Verification items for this drawing (mm, ordinates from the low corner). A direction names the side the tool comes from. Round coordinates to 2 decimals unless told otherwise and drop trailing zeros. Write each loop counter-clockwise with the first axis right and the second up, starting at its lowest first coordinate (ties: lowest second). Pieces come first, ordered by that corner, then holes. Notation, with made-up numbers: (52, 4.5) -> (88, 4.5) arc R35 ccw to (88, 37.5) -> close; hole circle Ø7 at (55.5, 24). An arc over 180 degrees is marked (long way). One line per question, with ' | ' between items.
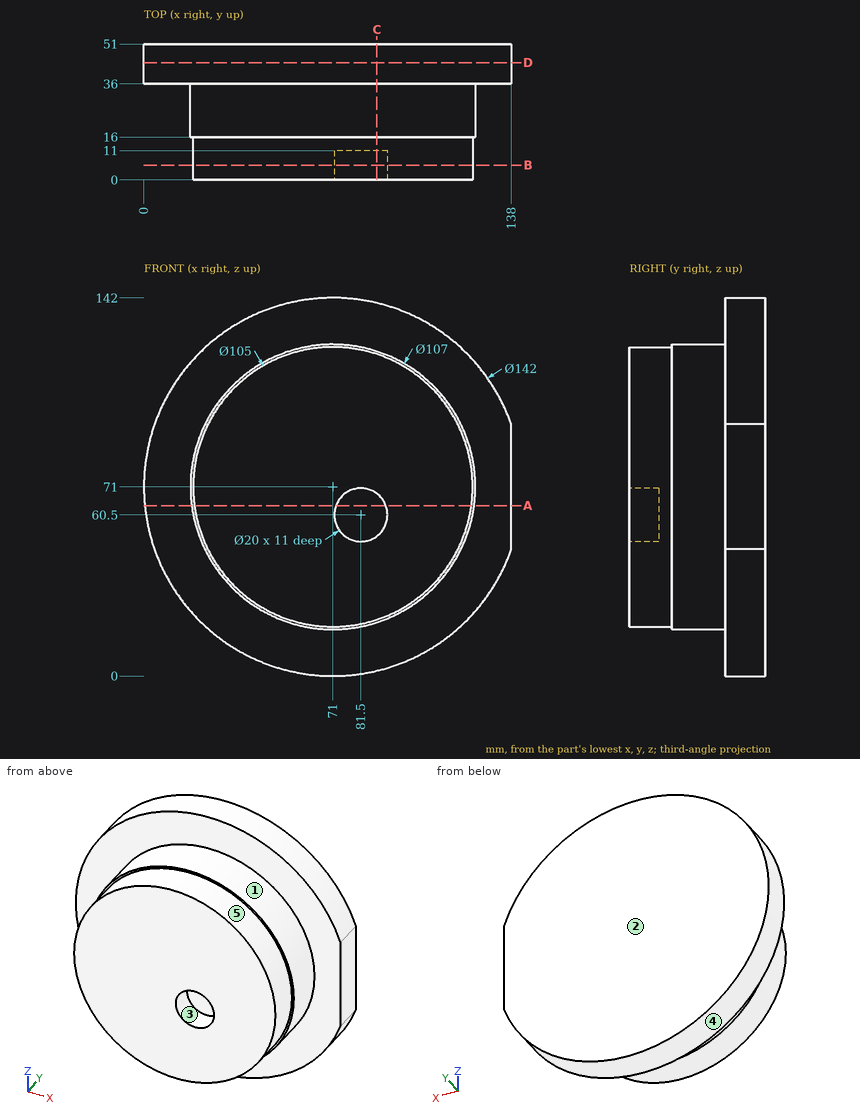
(1) Sectioned sample at A-A on z = 64. Record the cut outline in (x, y).
Resolved:
outline: (0.35, 36) -> (17.96, 36) -> (17.96, 16) -> (18.97, 16) -> (18.97, 0) -> (72.13, 0) -> (72.13, 11) -> (90.87, 11) -> (90.87, 0) -> (123.03, 0) -> (123.03, 16) -> (124.04, 16) -> (124.04, 36) -> (138, 36) -> (138, 51) -> (0.35, 51) -> close
(2) Material ranges on line 1 (X direction, y = 6.75, z = 60.5); line 2 (Y direction, x = 59, z = 6); line 3 (Z direction, x = 81.5, y = 2.5), recorded low to high.
Resolved:
line 1: x = 19.56 to 71.5, 91.5 to 122.44 | line 2: y = 36 to 51 | line 3: z = 19.56 to 50.5, 70.5 to 122.44
(3) Draft check along Z on the marked faces 1, 2 and 3. Enter one of: +Z half, -Z half, draft (parallel to the pull), parting line (faces both ways), or undercut.
Resolved:
face 1: parting line | face 2: draft | face 3: undercut
(4) Sectioned sample at D-D on y = 44. Record the cut outline in (x, z), then the cut area to 3 significant figures.
Resolved:
outline: (138, 47.51) -> (138, 94.49) arc R71 ccw (long way) to start | area: 15,700 mm2
(5) Go/stop test with flat-tipped pins: pin 1 (3 mm diameter, centred on x = 57.5, y = 35.5, fed in from +Z); pin 2 (10 mm diameter, centred on x = 31.5, y = 7, fed in from -Z); pin 3 (12 mm diameter, centred on y = 20, z = 32, fed in from +X). Record where each tip stops, or that it passes through.
Resolved:
pin 1: stops at z = 140.96 | pin 2: stops at z = 31.43 | pin 3: stops at x = 113.11
(6) Sectioned sample at B-B on y = 5.5. Record the cut outline in (x, z).
Resolved:
outline: circle Ø105 at (71, 71); hole circle Ø20 at (81.5, 60.5)
(7) Access from +Z, -Z, +X, -X, +Y, -Y to the whole of each face (thin tool, end or side, straight path). Record for the marked faces 4 and 5.
Resolved:
face 4: +Y, -Y | face 5: -Y
(8) Sectioned sample at C-C on x = 87.5. Record the cut outline in (y, z), then the cut area to 3 significant figures.
Resolved:
outline: (0, 21.16) -> (16, 21.16) -> (16, 20.11) -> (36, 20.11) -> (36, 1.94) -> (51, 1.94) -> (51, 140.06) -> (36, 140.06) -> (36, 121.89) -> (16, 121.89) -> (16, 120.84) -> (0, 120.84) -> (0, 68.5) -> (11, 68.5) -> (11, 52.5) -> (0, 52.5) -> close | area: 5,530 mm2
